Read the model definition and answer for the solid it produces. Units are mm, in the model's axes. Face numbers are marked on the shaded views. A direction names the side the tool comes from. Round coordinates to 2 decimals unless told otherwise and drop trailing zeros. Loops run counter-clockwise (first coordinate to the right, second up) from the corner with the lowest first, then second, coordinate; pieces in that order, holes last. Notation, with made-up numbers: (-33.75, 44.5) - (9.25, 44.5) arc R20 ccw to (9.25, 66.5) - close; hole circle Ø6 at (-30, 39). An arc over 180 degrees is marked (long way). Use CSV: the item, a comma, the result in double quotes. Start each with the question number.
1. Find section C-C (z = -7.75). Give the vertices of the cut face in (x, y).
2. Determine the mould class of the marked faces 1 and 2 for opening direction X: +X half, -X half, draft (parallel to the pull), parting line (faces both ways), or undercut.
3. Find section B-B (y = 0). Give the vertices of the cut face in (x, z).
4. Consider line 1 along Y through (x, z) = (0, -8); line 2 along Z through (x, y) = (9, 3.25); line 3 along Z through (x, y) = (-2.75, 5.75). Determine where each line is inside the solid, lowest interval first.
5. Given pin 1 Ø1.5 at (x, y) = (-1.5, 2.5) entering from +Z; pin 2 Ø12 at (x, y) = (5.5, 1.5) entering from +Z; pin 3 Ø1.5 at (x, z) = (2, -8) entering from -Y, each flat-ended and moving along its own axis, determine where each tip first touches the part or whether it passes through.
6. A tool of negligible diameter and unlimited length cuts with its end or side. For the marked faces 3 and 4, from which of +Z, -Z, +X, -X, +Y, -Y can it reach the whole face along a straight path? Write none if from no direction.
7. Find section A-A (x = 0). Give the vertices of the cut face in (y, z).
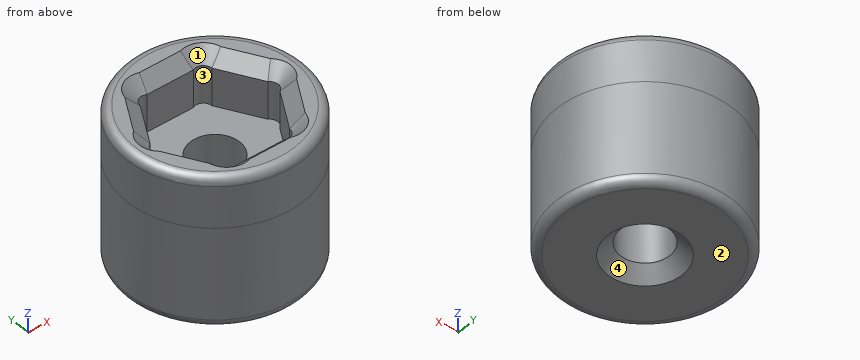
from build123d import *

# Parameters (mm, degrees)
SKETCH1_R           = 10.5
BOSS_EXTRUDE1_DEPTH = 6
BOSS_EXTRUDE2_START = 12
SKETCH2_R           = 10.5
SKETCH2_R_2         = 2.95
BOSS_EXTRUDE2_DEPTH = 12
CHAMFER1_SIZE       = 1.5
FILLET1_R           = 1


with BuildPart() as part:
    # Sketch1 → Boss-Extrude1 (new body)
    with BuildSketch(Plane.XY):
        Circle(SKETCH1_R)
        with BuildLine():
            Line((-2.75277675, 6.5), (2.75277675, 6.5))
            ThreePointArc((2.75277675, 6.5), (3.75277675, 6.5), (4.25277675, 5.633974596))
            Line((4.25277675, 5.633974596), (7.005553499, 0.866025404))
            ThreePointArc((7.005553499, 0.866025404), (7.505553499, 0), (7.005553499, -0.866025404))
            Line((7.005553499, -0.866025404), (4.25277675, -5.633974596))
            ThreePointArc((4.25277675, -5.633974596), (3.75277675, -6.5), (2.75277675, -6.5))
            Line((2.75277675, -6.5), (-2.75277675, -6.5))
            ThreePointArc((-2.75277675, -6.5), (-3.75277675, -6.5), (-4.25277675, -5.633974596))
            Line((-4.25277675, -5.633974596), (-7.005553499, -0.866025404))
            ThreePointArc((-7.005553499, -0.866025404), (-7.505553499, 0), (-7.005553499, 0.866025404))
            Line((-7.005553499, 0.866025404), (-4.25277675, 5.633974596))
            ThreePointArc((-4.25277675, 5.633974596), (-3.75277675, 6.5), (-2.75277675, 6.5))
        make_face(mode=Mode.SUBTRACT)
    extrude(amount=BOSS_EXTRUDE1_DEPTH)

    # Sketch2 → Boss-Extrude2 (add)
    with BuildSketch(Plane(origin=(0, 0, 0), x_dir=(-1, 0, 0), z_dir=(0, 0, -1)).offset(BOSS_EXTRUDE2_START)):
        Circle(SKETCH2_R)
        Circle(SKETCH2_R_2, mode=Mode.SUBTRACT)
    extrude(amount=-BOSS_EXTRUDE2_DEPTH)

    # Chamfer1
    chamfer1_edges = [part.edges().sort_by_distance(p)[0] for p in [
        (-3.75277675, 6.5, 6),
        (-5.629165125, 3.25, 6),
        (-7.505553499, 0, 6),
        (-5.629165125, -3.25, 6),
        (-3.75277675, -6.5, 6),
        (0, -6.5, 6),
        (3.75277675, -6.5, 6),
        (5.629165125, -3.25, 6),
        (7.505553499, 0, 6),
        (5.629165125, 3.25, 6),
        (3.75277675, 6.5, 6),
        (0, 6.5, 6),
        (2.95, 0, -12),
    ]]
    chamfer(chamfer1_edges, length=CHAMFER1_SIZE)

    # Fillet1
    fillet1_edges = [part.edges().sort_by_distance(p)[0] for p in [
        (-10.5, 0, 6),
        (10.5, 0, -12),
    ]]
    fillet(fillet1_edges, radius=FILLET1_R)


solid = part.part
Filled sheet:
1,outline,"circle Ø21 at (0, 0); hole circle Ø5.9 at (0, 0)"
2,face 1,"undercut"
2,face 2,"draft"
3,outline,"(-10.5, -11) arc R1 ccw to (-9.5, -12) - (-4.45, -12) - (-2.95, -10.5) - (-2.95, 0) - (-7.51, 0) - (-7.51, 4.5) - (-9.01, 6) - (-9.5, 6) arc R1 ccw to (-10.5, 5) - close; (2.95, -10.5) - (4.45, -12) - (9.5, -12) arc R1 ccw to (10.5, -11) - (10.5, 5) arc R1 ccw to (9.5, 6) - (9.01, 6) - (7.51, 4.5) - (7.51, 0) - (2.95, 0) - close"
4,line 1,"y = -10.5 to -2.95, 2.95 to 10.5"
4,line 2,"z = -12 to 6"
4,line 3,"z = -12 to 0"
5,pin 1,"stops at z = 0"
5,pin 2,"stops at z = 6"
5,pin 3,"stops at y = -10.43"
6,face 3,"+Z"
6,face 4,"-Z"
7,outline,"(-10.5, -11) arc R1 ccw to (-9.5, -12) - (-4.45, -12) - (-2.95, -10.5) - (-2.95, 0) - (-6.5, 0) - (-6.5, 4.5) - (-8, 6) - (-9.5, 6) arc R1 ccw to (-10.5, 5) - close; (2.95, -10.5) - (4.45, -12) - (9.5, -12) arc R1 ccw to (10.5, -11) - (10.5, 5) arc R1 ccw to (9.5, 6) - (8, 6) - (6.5, 4.5) - (6.5, 0) - (2.95, 0) - close"
